from build123d import *

# Parameters (mm, degrees)
SKETCH3_W           = 38.1
SKETCH3_H           = 6.35
BOSS_EXTRUDE1_DEPTH = 5.08
SKETCH4_R           = 1.905
CUT_EXTRUDE1_DEPTH  = 39.958168591
FILLET2_R           = 5.08


with BuildPart() as part:
    # Sketch3 → Boss-Extrude1 (new body)
    with BuildSketch(Plane(origin=(0, 0, 0), x_dir=(0, 1, 0), z_dir=(0, 0, 1))):
        with Locations((19.05, 3.175)):
            Rectangle(SKETCH3_W, SKETCH3_H)
    extrude(amount=BOSS_EXTRUDE1_DEPTH)

    # Sketch4 → Cut-Extrude1 (cut, through all)
    with BuildSketch(Plane(origin=(0, 0, 5.08), x_dir=(0, -1, 0), z_dir=(0, 0, 1))):
        with Locations(Location((-3.81, -3.175, 0), (0, 0, 90))):
            Circle(SKETCH4_R)
        with Locations(Location((-19.05, -3.175, 0), (0, 0, 90))):
            Circle(SKETCH4_R)
        with Locations(Location((-34.29, -3.175, 0), (0, 0, 90))):
            Circle(SKETCH4_R)
    extrude(amount=-CUT_EXTRUDE1_DEPTH, mode=Mode.SUBTRACT)

    # Fillet2
    # the kernel refuses this fillet: 5.08 mm, written as the material it takes off along each edge
    with BuildSketch(Plane(origin=(0, 38.1, -12.7), x_dir=(0, -1, 0), z_dir=(0, 0, 1)), Plane(origin=(-6.35, 38.1, -12.7), x_dir=(1, 0, 0), z_dir=(0, 0, 1))) as fillet2_piece_1:
        with BuildLine():
            CenterArc((FILLET2_R, -FILLET2_R), FILLET2_R, 90, 90)
            Line((0, -FILLET2_R), (0, 0))
            Line((0, 0), (FILLET2_R, 0))
        make_face()
    extrude(amount=30.48, mode=Mode.SUBTRACT)
    with BuildSketch(Plane(origin=(0, 0, -12.7), x_dir=(0, 1, 0), z_dir=(0, 0, 1)), Plane(origin=(-6.35, 0, -12.7), x_dir=(1, 0, 0), z_dir=(0, 0, 1))) as fillet2_piece_2:
        with BuildLine():
            CenterArc((FILLET2_R, FILLET2_R), FILLET2_R, 180, 90)
            Line((0, FILLET2_R), (0, 0))
            Line((0, 0), (FILLET2_R, 0))
        make_face()
    extrude(amount=30.48, mode=Mode.SUBTRACT)


solid = part.part
Input: part model. Units: mm. Frame: model coordinates. Give positions to 0.01 mm unless a question says otherwise; leave off trailing zeros. Write each loop counter-clockwise with the first axis right and the second up, starting at its lowest first coordinate (ties: lowest second). Pieces come first, ordered by that corner, then holes. Notation, with made-up numbers: M 68.25,-4 L 96.25,-4 A12 cw 96.25,1 Z; hole C 61,-30 d1. An arc over 180 degrees is marked long. Write item = value, one per line. Start each with the question number.
1) Draft query along X for faces 1 (the cylindrical face through (-5.46, 35.89, 2.5)), 2 (the flat face through (-1, 19, 0)), 3 (the cylindrical face through (-0.89, 2.21, 2.5)), 4 (the cylindrical face through (-2.151, 5.416, 2.576)). Return one class per face: +X half, -X half, draft (parallel to the pull), parting line (faces both ways), or undercut.
2) Cut plane A-A on z = 1. Return the cut outline in (x, y) (3 decimals).
3) Cut plane D-D on y = 3.81. Return the cut outline in (x, z).
4) Cut plane C-C on x = -4.75. Return the cut outline in (y, z).
5) Cut plane B-B on y = 19.05. Return the cut outline in (x, z).
6) Material intervals for line 1 along Y through (x, z) = (-3.75, 3.7); line 2 along Y through (x, z) = (-4, 3.1); line 3 along X through (y, z) = (3.5, 3.25), sorted ascending. Write a range as [from, to].
Solved:
q1.face_1 = -X half
q1.face_2 = draft
q1.face_3 = +X half
q1.face_4 = undercut
q2.outline = M -6.35,5.08 A5.08 ccw -3.175,0.371 A5.08 ccw 0,5.08 L 0,33.02 A5.08 ccw -3.175,37.729 A5.08 ccw -6.35,33.02 Z; hole C -3.175,3.81 d3.81; hole C -3.175,19.05 d3.81; hole C -3.175,34.29 d3.81
q3.outline = M -6.19,0 L -5.08,0 L -5.08,5.08 L -6.19,5.08 Z; M -1.27,0 L -0.16,0 L -0.16,5.08 L -1.27,5.08 Z
q4.outline = M 1.38,0 L 2.74,0 L 2.74,5.08 L 1.38,5.08 Z; M 4.88,0 L 17.98,0 L 17.98,5.08 L 4.88,5.08 Z; M 20.12,0 L 33.22,0 L 33.22,5.08 L 20.12,5.08 Z; M 35.36,0 L 36.72,0 L 36.72,5.08 L 35.36,5.08 Z
q5.outline = M -6.35,0 L -5.08,0 L -5.08,5.08 L -6.35,5.08 Z; M -1.27,0 L 0,0 L 0,5.08 L -1.27,5.08 Z
q6.line_1 = [0.65, 1.99], [5.63, 17.23], [20.87, 32.47], [36.11, 37.45]
q6.line_2 = [0.8, 2.09], [5.53, 17.33], [20.77, 32.57], [36.01, 37.3]
q6.line_3 = [-6.1, -5.05], [-1.3, -0.25]
